Geometry check sheet. Reference: drawing and pictorial views, mm from the part's lowest x, y, z. Give positions to 0.01 mm unless a question says otherwise; leave off trailing zeros. Write each loop counter-clockwise with the first axis right and the second up, starting at its lowest first coordinate (ties: lowest second). Pieces come first, ordered by that corner, then holes. Notation, with made-up numbers: (-33.75, 50) -> (6.25, 50) arc R20 ccw to (6.25, 74) -> close; hole circle Ø10 at (53.25, -14). An arc over 180 degrees is marked (long way). Write each question's results on one line, items separated by ' | '. Start each with the question number.
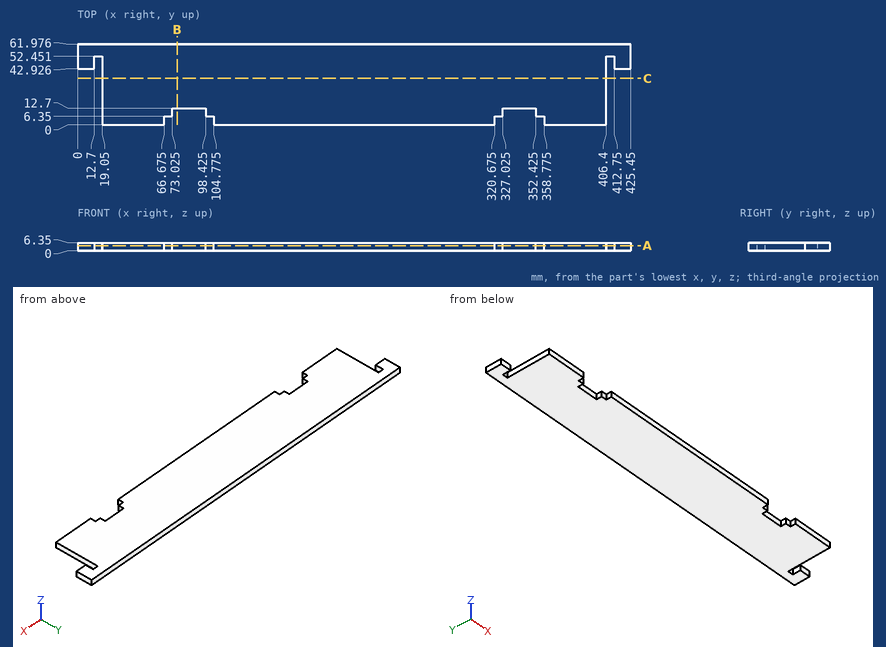
Item 1: Section check A-A on z = 4. Record the boundary of the cut face in (x, y) (3 decimals).
Item 2: Depth check by flat-ended pin: pin 1 Ø1 at (x, y) = (335, 31) entering from -Z; pin 2 Ø3 at (y, z) = (4.5, 3.5) entering from +X; pin 3 Ø3 at (x, z) = (409, 2) entering from -Y; pin 4 Ø1.5 at (y, z) = (14, 5.5) entering from -X. Enter the tip coordinate at first touch or a pass-through.
Item 3: Thickness scan on probe 1 along X at (y, z) = (47.5, 6.25); probe 2 along X at (y, z) = (11.5, 2) (3 decimals); probe 3 along X at (y, z) = (42, 4). Record the ranges inside material, lowest first. Write a range as from..to.
Item 4: Section check B-B on x = 76.5. Record the boundary of the cut face in (y, z).
Item 5: Section check C-C on y = 35.5. Record the boundary of the cut face in (x, z), then the cut area to 3 significant figures.
Check sheet entries:
1) outline: (0, 42.926) -> (12.7, 42.926) -> (12.7, 52.451) -> (19.05, 52.451) -> (19.05, 0) -> (66.675, 0) -> (66.675, 6.35) -> (73.025, 6.35) -> (73.025, 12.7) -> (98.425, 12.7) -> (98.425, 6.35) -> (104.775, 6.35) -> (104.775, 0) -> (320.675, 0) -> (320.675, 6.35) -> (327.025, 6.35) -> (327.025, 12.7) -> (352.425, 12.7) -> (352.425, 6.35) -> (358.775, 6.35) -> (358.775, 0) -> (406.4, 0) -> (406.4, 52.451) -> (412.75, 52.451) -> (412.75, 42.926) -> (425.45, 42.926) -> (425.45, 61.976) -> (0, 61.976) -> close
2) pin 1: stops at z = 0 | pin 2: stops at x = 406.4 | pin 3: stops at y = 52.45 | pin 4: stops at x = 19.05
3) probe 1: x = 0..12.7, 19.05..406.4, 412.75..425.45 | probe 2: x = 19.05..73.025, 98.425..327.025, 352.425..406.4 | probe 3: x = 19.05..406.4
4) outline: (12.7, 0) -> (61.98, 0) -> (61.98, 6.35) -> (12.7, 6.35) -> close
5) outline: (19.05, 0) -> (406.4, 0) -> (406.4, 6.35) -> (19.05, 6.35) -> close | area: 2,460 mm^2
